The model under review builds one solid part; all positions refer to its coordinate system, in mm. A direction names the side the tool comes from. Round coordinates to 2 decimals unless told otherwise and drop trailing zeros. Loops run counter-clockwise (first coordinate to the right, second up) from the corner with the lowest first, then second, coordinate; pieces in that order, holes last. Notation, with made-up numbers: (-9, 60) -> (22, 60) arc R27 cw to (22, 97) -> close; hole circle Ø4 at (5, 71). An arc over 180 degrees is marked (long way). Use CSV: the item, a comma, the result in double quotes. Start each with the question number.
```python
from build123d import *

# Parameters (mm, degrees)
BOX_W        = 31
BOX_H        = 21
BOX_DEPTH    = 10
PAD_DEPTH    = 20
SKETCH002_R  = 2.5
POCKET_DEPTH = 7.001


with BuildPart() as cubo:
    # Box → Box (new body)
    with BuildSketch(Plane(origin=(-15, -10, 1), x_dir=(1, 0, 0), z_dir=(0, 0, 1))):
        with Locations((15.5, 10.5)):
            Rectangle(BOX_W, BOX_H)
    extrude(amount=BOX_DEPTH)


with BuildPart() as pocket:
    # Sketch → Pad (new body, symmetric)
    with BuildSketch(Plane.XZ):
        Polygon((-25, -15), (-10, -15), (-5, 7), (5, 7), (10, -15), (25, -15), (25, -8), (15, -8), (10, 15), (-10, 15), (-15, -8), (-25, -8), align=None)
    extrude(amount=PAD_DEPTH, both=True)

    # Cut: cut Cubo
    add(cubo.part, mode=Mode.SUBTRACT)

    # Sketch002 → Pocket (cut, through all)
    with BuildSketch(Plane.XY.offset(-8)):
        with Locations((-20.002137, 12)):
            Circle(SKETCH002_R)
        with Locations((-20.002137, -12)):
            Circle(SKETCH002_R)
        with Locations((19.997863, 12)):
            Circle(SKETCH002_R)
        with Locations((19.997863, -12)):
            Circle(SKETCH002_R)
    extrude(amount=-POCKET_DEPTH, mode=Mode.SUBTRACT)


solid = pocket.part
```
1. Take a section at A-A, the plane y = 12. Give the boundary of the cut face in (x, z).
2. For line 1 along Y through (x, z) = (-6, 9); line 2 along Z through (x, y) = (-0.5, 14); line 3 along Z through (x, y) = (-20, -4), list the stretches that pass through material, from the lowest coordinate up. Write a range as from..to.
3. Take a section at D-D, the plane z = 2.75. Give the boundary of the cut face in (x, y).
4. Take a section at B-B, the plane z = -3.75. Give the boundary of the cut face in (x, y).
5. The part is to be moulded in two halves that separate along Y. For faces 1 (the face through (20, 0, -8)), 2 (the face through (10, 1, 1)), 3 (the face through (-6, 20, 4)), say which applies: pulls with the +Y half, pulls with the -Y half, needs draft (parallel to the pull), parting line crosses it, or undercut.
6. Take a section at C-C, the plane x = -1.5. Give the boundary of the cut face in (y, z).
7. Clearance check with flat-ended pins moving along their axes: P1, Ø6.5, axis at x = -20, y = 12, coming from the +Z side; P2, Ø2, axis at y = -11.5, z = -6, coming from the -X side; P3, Ø2.5, axis at x = 0, y = 16.5, coming from the -Z side. State where each tip first meets the part, or that it passes through.
8. For faces 4 (the face through (-20.54, -14.44, -11.45)), 5 (the face through (0, 1, 11)), 6 (the face through (-20, 0, -8)), 7 (the face through (8.02, -0.28, -6.29)), list the 3-axis set-ups (+Z, -Z, +X, -X, +Y, -Y) from which the entire face can be reached by the end or side of a thin tool; tool diameter is ignored.
Results:
1,outline,"(-25, -15) -> (-22.5, -15) -> (-22.5, -8) -> (-25, -8) -> close; (-17.5, -15) -> (-10, -15) -> (-5, 7) -> (5, 7) -> (10, -15) -> (17.5, -15) -> (17.5, -8) -> (15, -8) -> (10, 15) -> (-10, 15) -> (-15, -8) -> (-17.5, -8) -> close; (22.5, -15) -> (25, -15) -> (25, -8) -> (22.5, -8) -> close"
2,line 1,"-20..-10, 11..20"
2,line 2,"7..15"
2,line 3,"-15..-8"
3,outline,"(-12.66, -20) -> (-5.97, -20) -> (-5.97, -10) -> (-12.66, -10) -> close; (-12.66, 11) -> (-5.97, 11) -> (-5.97, 20) -> (-12.66, 20) -> close; (5.97, -20) -> (12.66, -20) -> (12.66, -10) -> (5.97, -10) -> close; (5.97, 11) -> (12.66, 11) -> (12.66, 20) -> (5.97, 20) -> close"
4,outline,"(-14.08, -20) -> (-7.44, -20) -> (-7.44, 20) -> (-14.08, 20) -> close; (7.44, -20) -> (14.08, -20) -> (14.08, 20) -> (7.44, 20) -> close"
5,face 1,"needs draft"
5,face 2,"undercut"
5,face 3,"pulls with the +Y half"
6,outline,"(-20, 7) -> (-10, 7) -> (-10, 11) -> (11, 11) -> (11, 7) -> (20, 7) -> (20, 15) -> (-20, 15) -> close"
7,P1,"z = -8"
7,P2,"x = -14.78"
7,P3,"z = 7"
8,face 4,"+Z, -Z"
8,face 5,"+X, -X"
8,face 6,"+Z, -X, +Y, -Y"
8,face 7,"-Z, +Y, -Y"
